from build123d import *

# Parameters (mm, degrees)
SKETCH1_W           = 75.1
SKETCH1_H           = 5
SKETCH1_R           = 0.7
SKETCH1_R_2         = 0.5
BOSS_EXTRUDE1_DEPTH = 4
BOSS_EXTRUDE2_DEPTH = 5
SKETCH4_R           = 0.5
CUT_EXTRUDE1_DEPTH  = 33
SKETCH5_R           = 0.702970984
CUT_EXTRUDE2_DEPTH  = 10


with BuildPart() as part:
    # Sketch1 → Boss-Extrude1 (new body)
    with BuildSketch(Plane(origin=(0, 0, 0), x_dir=(1, 0, 0), z_dir=(0, 1, 0))):
        Rectangle(SKETCH1_W, SKETCH1_H)
        with Locations(Location((-33.405, 0, 0), (0, 0, 270))):
            Circle(SKETCH1_R, mode=Mode.SUBTRACT)
        with Locations(Location((33.405, 0, 0), (0, 0, 270))):
            Circle(SKETCH1_R, mode=Mode.SUBTRACT)
        with Locations(Location((0, 0, 0), (0, 0, 270))):
            Circle(SKETCH1_R_2, mode=Mode.SUBTRACT)
    extrude(amount=BOSS_EXTRUDE1_DEPTH)

    # Sketch3 → Boss-Extrude2 (add)
    with BuildSketch(Plane.XY.offset(2.5)):
        with BuildLine():
            Line((-13.101977393, 4), (12.898022607, 4))
            ThreePointArc((12.898022607, 4), (5.892969188, 6.964559048), (3, 13.999480017))
            Line((3, 13.999480017), (3, 19))
            ThreePointArc((3, 19), (2.414213562, 20.414213562), (1, 21))
            Line((1, 21), (-1.101977393, 21))
            ThreePointArc((-1.101977393, 21), (-2.516190955, 20.414213562), (-3.101977393, 19))
            Line((-3.101977393, 19), (-3.101977393, 14))
            ThreePointArc((-3.101977393, 14), (-6.030909581, 6.928932188), (-13.101977393, 4))
        make_face()
    extrude(amount=-BOSS_EXTRUDE2_DEPTH)

    # Sketch4 → Cut-Extrude1 (cut)
    with BuildSketch(Plane.XZ):
        with Locations(Location((0, 0, 0), (0, 0, 90))):
            Circle(SKETCH4_R)
    extrude(amount=-CUT_EXTRUDE1_DEPTH, mode=Mode.SUBTRACT)

    # Sketch5 → Cut-Extrude2 (cut)
    with BuildSketch(Plane.XY.offset(2.5)):
        with Locations((-0.101977393, 18)):
            Circle(SKETCH5_R)
    extrude(amount=-CUT_EXTRUDE2_DEPTH, mode=Mode.SUBTRACT)


solid = part.part
Part model, mm, in its own coordinate system. A direction names the side the tool comes from. Coordinates: 2 decimals unless noted, no trailing zeros. Order: outer loops, then holes, each group sorted by start corner. A loop starts at its lowest first (then second) coordinate and runs counter-clockwise, first axis right, second up.
(1) Slice it at C-C, the plane x = -21.5. Write the cut outline in (y, z).
Check sheet entries:
outline: (0, -2.5) - (4, -2.5) - (4, 2.5) - (0, 2.5) - close
(2) Slice it at A-A, the plane z = 1.45. Write the cut outline in (x, y).
Check sheet entries:
outline: (-37.55, 0) - (37.55, 0) - (37.55, 4) - (12.9, 4) arc R10 cw to (3, 14) - (3, 19) arc R2 ccw to (1, 21) - (-1.1, 21) arc R2 ccw to (-3.1, 19) - (-3.1, 14) arc R10 cw to (-13.1, 4) - (-37.55, 4) - close; hole circle Ø1.41 at (-0.1, 18)
(3) Slice it at D-D, the plane y = 4.75. Write the cut outline in (x, z).
Check sheet entries:
outline: (-9.3, -2.5) - (9.2, -2.5) - (9.2, 2.5) - (-9.3, 2.5) - close; hole circle Ø1 at (0, 0)
(4) Probe L1, parallel to X at y = 2.6, z = 0 (3 decimals); L2, parallel to X at y = 16.75, z = 1.3; L3, parallel to X at y = 16, z = 0.1. List the from-to ranges inside material, lowest first.
Check sheet entries:
L1: x = -37.55 to -34.105, -32.705 to -0.5, 0.5 to 32.705, 34.105 to 37.55
L2: x = -3.1 to 3
L3: x = -3.1 to -0.49, 0.49 to 3
(5) Pin check, flat tips, straight feed: pin 1 Ø2.5 at (x, z) = (26, 1) entering from +Y; pin 2 Ø1.5 at (y, z) = (7, -0.5) entering from +X; pin 3 Ø1.8 at (x, y) = (-0.1, 18) entering from -Z; pin 4 Ø1.1 at (x, z) = (-33.405, 0) entering from -Y. Stop position of each tip, or through.
Check sheet entries:
pin 1: stops at y = 4
pin 2: stops at x = 6.68
pin 3: stops at z = -2.5
pin 4: passes through
(6) Pull direction Y, two halves, no side cores. Call faces 1 (the face through (-1, 0, 0)), 2 (the face through (-0.804, 18.031, 0.035)), 3 (the face through (32.72, 1.97, -0.15)), 4 (the face through (-25, 4, 0)): pulls with the +Y half, pulls with the -Y half, needs draft (parallel to the pull), parting line crosses it, or undercut.
Check sheet entries:
face 1: pulls with the -Y half
face 2: undercut
face 3: needs draft
face 4: pulls with the +Y half
(7) Tool access for faces 5 (the face through (0, 5, 2.5)), 6 (the face through (3, 16, 0)), 7 (the face through (-3.102, 17, 0)): list every direction of +Z, -Z, +X, -X, +Y, -Y with a clear straight run to the whole face (end or side of a thin tool).
Check sheet entries:
face 5: +Z, +X, -X, +Y, -Y
face 6: +Z, -Z, +X, +Y
face 7: +Z, -Z, -X, +Y
(8) Slice it at B-B, the plane y = 14.75. Write the cut outline in (x, z).
Check sheet entries:
outline: (-3.1, -2.5) - (3, -2.5) - (3, 2.5) - (-3.1, 2.5) - close; hole circle Ø1 at (0, 0)
